from build123d import *

# Parameters (mm, degrees)
F0_W     = 50.4226610065
F0_H     = 50.1393936574
F1_DEPTH = 45
F2_T     = -5
F3_W     = 9.6008158289
F3_H     = 5
F4_DEPTH = 0.5
F6_D     = 1
F6_DEPTH = 2
F6_TIP   = 0.3004303095
F7_R     = 5


with BuildPart() as f1:
    # F0 (on Top) → F1 (new body)
    with BuildSketch(Plane.XY):
        Rectangle(F0_W, F0_H)
    extrude(amount=F1_DEPTH)

    # F2
    f2_openings = [f1.faces().sort_by_distance(p)[0] for p in [
        (0, 0, 45),
    ]]
    offset(amount=F2_T, openings=f2_openings)

    # F3 (on face) → F4 (cut)
    with BuildSketch(Plane.XY.offset(45)):
        with Locations((-12.5397194643, -22.5696968287)):
            Rectangle(F3_W, F3_H)
    extrude(amount=-F4_DEPTH, mode=Mode.SUBTRACT)

    # F6 (one way)
    with BuildSketch(Plane.XY.offset(44.5)):
        with Locations((-12.7751557156, -22.5923974067), (12.2276665643, -22.5696968287)):
            Circle(F6_D / 2)
    extrude(amount=-F6_DEPTH, mode=Mode.SUBTRACT)
    with Locations(Plane.XY.offset(44.5)):
        with Locations((-12.7751557156, -22.5923974067), (12.2276665643, -22.5696968287)):
            with Locations((0, 0, -(F6_DEPTH + F6_TIP / 2))):  # 118° drill point
                Cone(0, F6_D / 2, F6_TIP, mode=Mode.SUBTRACT)

    # F7
    f7_edges = [f1.edges().sort_by_distance(p)[0] for p in [
        (25.211331, -25.069697, 22.5),
        (-25.211331, -25.069697, 22.5),
        (-25.211331, 25.069697, 22.5),
        (25.211331, 25.069697, 22.5),
    ]]
    fillet(f7_edges, radius=F7_R)


solid = f1.part
Geometry check sheet. Reference: the model listing, model coordinates, mm. A direction names the side the tool comes from. Round coordinates to 2 decimals unless told otherwise and drop trailing zeros. Write each loop counter-clockwise with the first axis right and the second up, starting at its lowest first coordinate (ties: lowest second). Pieces come first, ordered by that corner, then holes. Notation, with made-up numbers: (5.25, -22) - (41.25, -22) arc R22 cw to (41.25, -10) - close; hole circle Ø4 at (74, 16.25). An arc over 180 degrees is marked (long way). One line per item, written item: value.
1. Scan lines: L1, parallel to Y at x = 15.5, z = 40.5; L2, parallel to X at y = 15.5, z = 10.5; L3, parallel to Z at x = 6.5, y = 0.5. Record each from-to range of solid material in increasing order.
The answers:
L1: y = -25.07 to -20.07, 20.07 to 25.07
L2: x = -25.21 to -20.21, 20.21 to 25.21
L3: z = 0 to 5
2. Cross-section at A-A on z = 24. Record the boundary of the cut face in (x, y), and give its area (3 significant figures).
The answers:
outline: (-25.21, -20.07) arc R5 ccw to (-20.21, -25.07) - (20.21, -25.07) arc R5 ccw to (25.21, -20.07) - (25.21, 20.07) arc R5 ccw to (20.21, 25.07) - (-20.21, 25.07) arc R5 ccw to (-25.21, 20.07) - close; hole (-20.21, -20.07) - (20.21, -20.07) - (20.21, 20.07) - (-20.21, 20.07) - close
area: 884 mm^2
3. Mould release check, pull along X, two halves, no side actions. Record for faces 4 (the face through (0, 25.07, 22)), 5 (the face through (23.71, -23.64, 22.82)), 6 (the face through (0, 0, 5)): released by +X, released by -X, zero draft, split by the parting line, or undercut.
The answers:
face 4: zero draft
face 5: released by +X
face 6: undercut
4. Set-up check for faces 1 (the face through (-20.211, 0, 25)), 2 (the face through (-14, -23, 44.5)), 3 (the face through (23.71, 23.64, 22.82)): record each of +Z, -Z, +X, -X, +Y, -Y from which the full face is reachable in a straight line by a thin tool's end or side.
The answers:
face 1: +Z
face 2: +Z, -Y
face 3: +Z, -Z, +X, +Y
5. Cross-section at C-C on y = 5.5. Record the boundary of the cut face in (x, z), and give its area (3 significant figures).
The answers:
outline: (-25.21, 0) - (25.21, 0) - (25.21, 45) - (20.21, 45) - (20.21, 5) - (-20.21, 5) - (-20.21, 45) - (-25.21, 45) - close
area: 652 mm^2
6. Cross-section at B-B on x = -10.5. Record the boundary of the cut face in (y, z).
The answers:
outline: (-25.07, 0) - (25.07, 0) - (25.07, 45) - (20.07, 45) - (20.07, 5) - (-20.07, 5) - (-20.07, 44.5) - (-25.07, 44.5) - close
7. Depth check by flat-ended pin: pin 1 Ø0.5 at (x, y) = (12.5, -22.5) entering from -Z; pin 2 Ø5.5 at (x, y) = (-13, -22) entering from +Z; pin 3 Ø3 at (x, y) = (1, 5) entering from +Z. Enter the tip coordinate at first touch or a pass-through.
The answers:
pin 1: stops at z = 0
pin 2: stops at z = 44.5
pin 3: stops at z = 5
